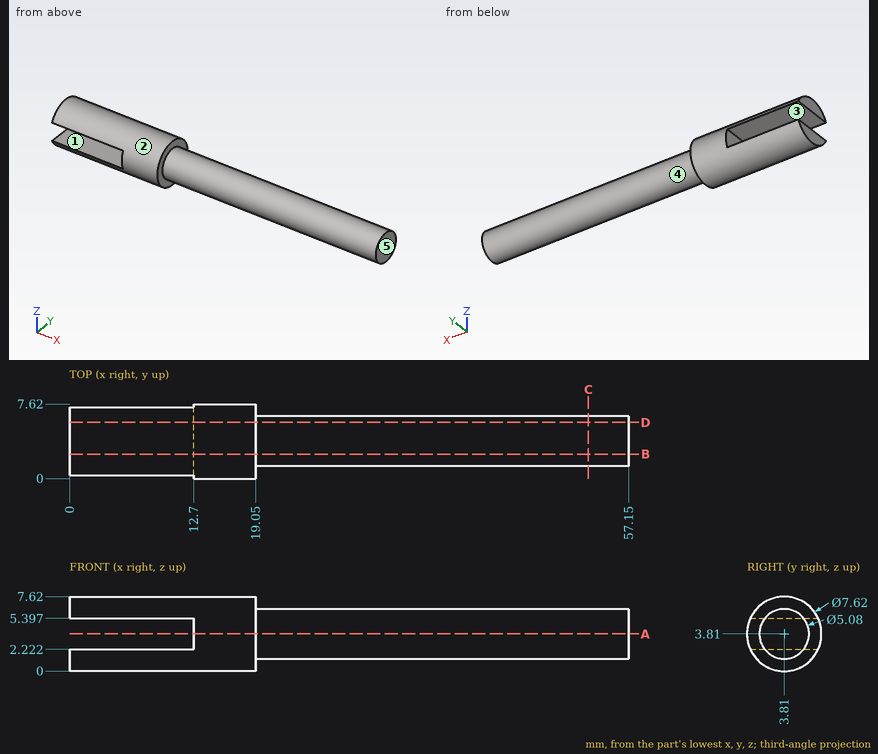
Part print with two shaded views. Sizes in mm from the minimum x, y, z corner. A direction names the side the tool comes from. Coordinates: 2 decimals unless noted, no trailing zeros. Loops run counter-clockwise (first coordinate to the right, second up) from the corner with the lowest first, then second, coordinate; pieces in that order, holes last. Notation, with made-up numbers: (-31.5, -16.75) -> (13.5, -16.75) arc R23 ccw to (13.5, 8.25) -> close; hole circle Ø5 at (2.5, 38.25). An arc over 180 degrees is marked (long way). Answer as a JSON object with one key per item and string values.
Q1. Pull direction Z, two halves, no side cores. Call the marked faces 3, 4 and 5: released by +Z, released by -Z, zero draft, split by the parting line, or undercut.
Report:
{"face 3": "undercut", "face 4": "split by the parting line", "face 5": "zero draft"}
Q2. Cut at A-A (z = 3.81). List the corners of the cut face in (x, y).
Report:
{"outline": "(12.7, 0) -> (19.05, 0) -> (19.05, 1.27) -> (57.15, 1.27) -> (57.15, 6.35) -> (19.05, 6.35) -> (19.05, 7.62) -> (12.7, 7.62) -> close"}
Q3. Probe probe 1 along X at (y, z) = (2.5, 4.5); probe 2 along Z at (x, y) = (5, 6.25) (1 decimal); probe 3 along X at (y, z) = (5.5, 7). List the from-to ranges inside material, lowest first.
Report:
{"probe 1": "x = 12.7 to 57.15", "probe 2": "z = 0.9 to 2.2, 5.4 to 6.7", "probe 3": "x = 0 to 19.05"}
Q4. Cut at D-D (y = 5.75). List the corners of the cut face in (x, z).
Report:
{"outline": "(0, 0.53) -> (19.05, 0.53) -> (19.05, 2.17) -> (57.15, 2.17) -> (57.15, 5.45) -> (19.05, 5.45) -> (19.05, 7.09) -> (0, 7.09) -> (0, 5.4) -> (12.7, 5.4) -> (12.7, 2.22) -> (0, 2.22) -> close"}
Q5. Flat gauge pins, fed straight in: P1, Ø1.5, axis at x = 36.5, z = 2.5, coming from the +Y side; P2, Ø4, axis at x = 6, y = 6.5, coming from the +Z side; P3, Ø3, axis at x = 32, y = 2, coming from the -Z side. Where does each tip first touch, or does it go through?
Report:
{"P1": "stops at y = 6.29", "P2": "stops at z = 7.56", "P3": "stops at z = 1.29"}
Q6. 3-axis set-ups, long thin cutter, end or side, ignore diameter. For the marked faces 1 and 2: which of +Z, -Z, +X, -X, +Y, -Y reach the whole face in a straight line?
Report:
{"face 1": "-X, +Y, -Y", "face 2": "+X, -X"}
Q7. Cut at C-C (x = 53). List the corners of the cut face in (y, z), and give its area (3 significant figures).
Report:
{"outline": "circle Ø5.08 at (3.81, 3.81)", "area": "20.3 mm2"}
Q8. Cut at B-B (y = 2.5). List the corners of the cut face in (x, z), and give its area (3 significant figures).
Report:
{"outline": "(0, 0.23) -> (19.05, 0.23) -> (19.05, 1.63) -> (57.15, 1.63) -> (57.15, 5.99) -> (19.05, 5.99) -> (19.05, 7.39) -> (0, 7.39) -> (0, 5.4) -> (12.7, 5.4) -> (12.7, 2.22) -> (0, 2.22) -> close", "area": "262 mm2"}
